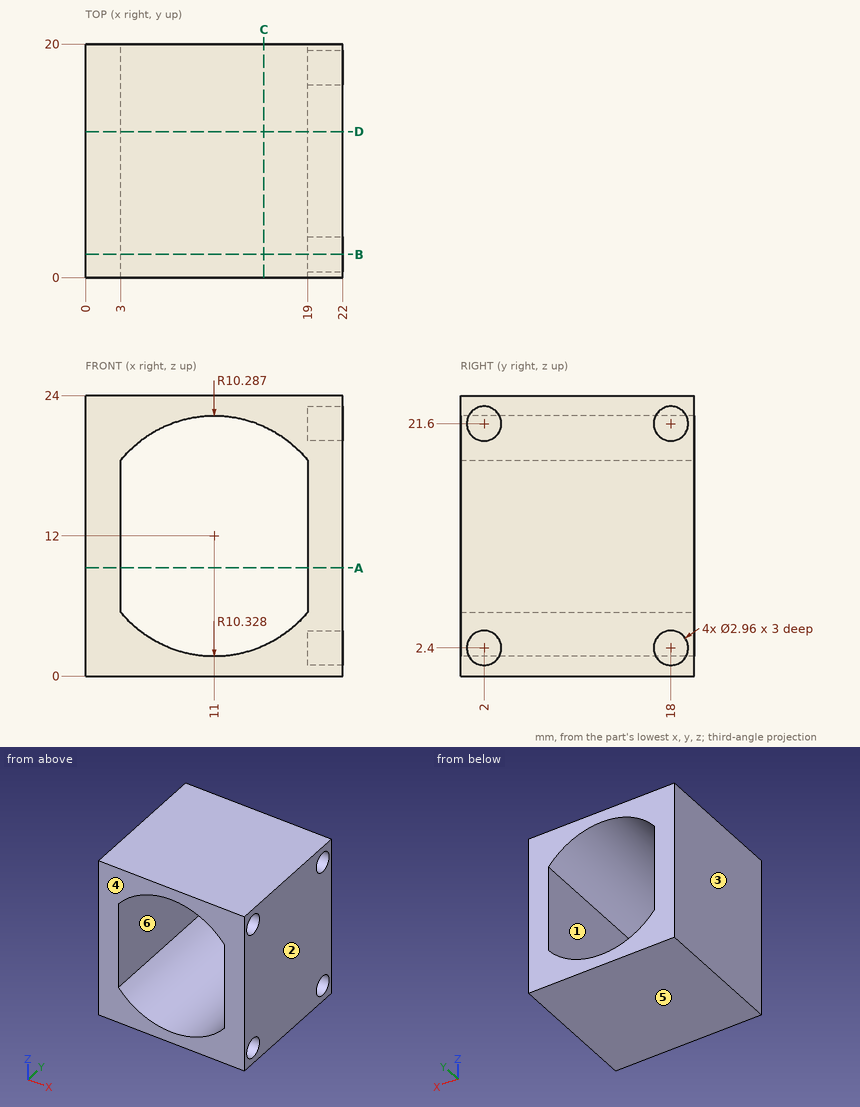
Can you work these out from the drawing? Everything is in mm from the part's minimum corner. A direction names the side the tool comes from. Give positions to 0.01 mm unless a question says otherwise; leave off trailing zeros. Order: outer loops, then holes, each group sorted by start corner. A loop starts at its lowest first (then second) coordinate and runs counter-clockwise, first axis right, second up. Notation, with made-up numbers: M -15,-37 L 32,-37 A33 cw 32,-5 Z; hole C 39.25,51 d3. An arc over 180 degrees is marked long. One line per item, written item: value.
Item 1: Please list where these lines run through material, in increasing order: line 1 (Y direction, x = 21.2, z = 21.6); line 2 (X direction, y = 12.5, z = 9); line 3 (Z direction, x = 7.5, y = 10.5).
Verdict:
line 1: 0 to 0.52, 3.48 to 16.52, 19.48 to 20
line 2: 0 to 3, 19 to 22
line 3: 0 to 2.28, 21.67 to 24
Item 2: If we section it at C-C on x = 15.25: Write out the boundary of the cut face in (y, z).
Verdict:
outline: M 0,0 L 20,0 L 20,2.59 L 0,2.59 Z; M 0,21.37 L 20,21.37 L 20,24 L 0,24 Z
Item 3: If we section it at D-D on y = 12.5: Write out the boundary of the cut face in (x, z) (1 decimal).
Verdict:
outline: M 0,0 L 22,0 L 22,24 L 0,24 Z; hole M 3,5.5 A10.3 ccw 19,5.5 L 19,18.5 A10.3 ccw 3,18.5 Z
Item 4: For the marked faces 5 and 6, which set-ups out of +Z, -Z, +X, -X, +Y, -Y let a thin tool reach every point of the face, with its end or its side?
Verdict:
face 5: -Z, +X, -X, +Y, -Y
face 6: +Y, -Y
Item 5: If we section it at B-B on y = 2: Write out the boundary of the cut face in (x, z) (1 decimal).
Verdict:
outline: M 0,0 L 22,0 L 22,0.9 L 19,0.9 L 19,3.9 L 22,3.9 L 22,20.1 L 19,20.1 L 19,23.1 L 22,23.1 L 22,24 L 0,24 Z; hole M 3,5.5 A10.3 ccw 19,5.5 L 19,18.5 A10.3 ccw 3,18.5 Z
Item 6: If we section it at A-A on z = 9.25: Write out the boundary of the cut face in (x, y), and give its area (3 significant figures).
Verdict:
outline: M 0,0 L 3,0 L 3,20 L 0,20 Z; M 19,0 L 22,0 L 22,20 L 19,20 Z
area: 120 mm2
Item 7: If we mould it in two halves opening along X, with no side actions, what happens to the marked faces 1, 2, 3 and 4? For each: pulls with the +X half, pulls with the -X half, needs draft (parallel to the pull), parting line crosses it, or undercut.
Verdict:
face 1: undercut
face 2: pulls with the +X half
face 3: pulls with the -X half
face 4: needs draft
Item 8: For pin 1 (10 mm diameter, centred on x = 9.5, z = 8.5, fed in from -Y); pin 2 (2.5 mm diameter, centred on y = 2, z = 2.4, fed in from +X), each with a flat end and sliding along its axis, tell me the tip position at first contact or that it passes through.
Verdict:
pin 1: through
pin 2: x = 19
